```python
from build123d import *

# Parameters (mm, degrees)
F1_DEPTH = 101.6
F2_R     = 2.54
F3_R     = 2.54
F4_R     = 2.54
F5_R     = 2.54
F7_D     = 1.9939


with BuildPart() as f1:
    # F0 (on Top) → F1 (new body)
    with BuildSketch(Plane.XY):
        Polygon((-25.4, 0), (0, 0), (25.4, 0), (25.4, 3.048), (22.6301808, 3.048), (22.6301808, 7.5232392634), (2.54, 7.5232392634), (2.54, 4.2931226644), (0, 4.2931226644), (-2.54, 4.2931226644), (-2.54, 7.5232392634), (-22.6301808, 7.5232392634), (-22.6301808, 3.048), (-25.4, 3.048), align=None)
    extrude(amount=F1_DEPTH)

    # F2
    f2_edges = [f1.edges().sort_by_distance(p)[0] for p in [
        (22.630181, 7.523239, 50.8),
    ]]
    fillet(f2_edges, radius=F2_R)

    # F3
    f3_edges = [f1.edges().sort_by_distance(p)[0] for p in [
        (22.630181, 3.048, 50.8),
    ]]
    fillet(f3_edges, radius=F3_R)

    # F4
    f4_edges = [f1.edges().sort_by_distance(p)[0] for p in [
        (-22.630181, 7.523239, 50.8),
    ]]
    fillet(f4_edges, radius=F4_R)

    # F5
    f5_edges = [f1.edges().sort_by_distance(p)[0] for p in [
        (-22.630181, 3.048, 50.8),
        (-22.630181, 4.983239, 50.8),
    ]]
    fillet(f5_edges, radius=F5_R)

    # F7 (through all)
    with Locations(Plane.XZ):
        with Locations((0, 81.2863707542), (0, 62.5548958778), (0, 40.594484657), (0, 18.223406747)):
            Hole(F7_D / 2)


solid = f1.part
```
Here's how the part is built. I have some questions about the finished solid (model axes, mm). A direction names the side the tool comes from. Give positions to 0.01 mm unless a question says otherwise; leave off trailing zeros. Order: outer loops, then holes, each group sorted by start corner. A loop starts at its lowest first (then second) coordinate and runs counter-clockwise, first axis right, second up. Notation, with made-up numbers: M 26.25,19.25 L 59.25,19.25 A15 ccw 59.25,33.25 Z; hole C 41.25,63.5 d6. An arc over 180 degrees is marked long. Use a Markdown table: item, result. Add a question column.
1. If we mould it in two halves opening along X, with no side actions, what happens to faces 3 (the flat face through (0, 0, 50)), 4 (the cylindrical face through (-21.757, 6.9, 51.511)), 5 (the cylindrical face through (21.795, 6.866, 51.511)), 6 (the cylindrical face through (0.216, 2.177, 61.582))? For each: +X half, -X half, draft (parallel to the pull), parting line (faces both ways), or undercut.
2. I need wall thicknesses on probe 1 along Z at (x, y) = (0, 1.8); probe 2 along Y at (x, z) = (-1.5, 65.5); probe 3 along X at (y, z) = (6, 61.5). Which ranges of each line are inside material? Lowest first, please. Write a range as from..to.
3. Suppose I cut it at B-B (y = 6.25). List the corners of the cut face in (x, z) for me, and give its area (3 significant figures).
4. Suppose I cut it at A-A (x = 0). List the corners of the cut face in (y, z) for me.
5. On a 3-axis mill with a long thin cutter (end or side, diameter ignored), from which of +Z, -Z, +X, -X, +Y, -Y can I reach the whole of each face in a straight line? I mean faces 1 (the cylindrical face through (0.22, 2.18, 17.25)), 2 (the flat face through (2.54, 6, 50)). Say none if no direction works.
6. For pin 1 Ø1.8 at (x, z) = (0, 62.55) entering from +Y; pin 2 Ø3 at (x, z) = (0, 81.29) entering from +Y; pin 3 Ø1 at (y, z) = (5, 36) entering from -X; pin 4 Ø1.6 at (y, z) = (5.5, 70.5) entering from +X, each with a flat end and sliding along its axis, tell me the tip position at first contact or that it passes through.
Results list:
| question | item | result |
|---|---|---|
| 1 | face 3 | draft |
| 1 | face 4 | -X half |
| 1 | face 5 | +X half |
| 1 | face 6 | undercut |
| 2 | probe 1 | z = 0..17.23, 19.22..39.6, 41.59..61.56, 63.55..80.29, 82.28..101.6 |
| 2 | probe 2 | y = 0..4.29 |
| 2 | probe 3 | x = -22.42..-2.54, 2.54..22.42 |
| 3 | outline | M -22.29,0 L -2.54,0 L -2.54,101.6 L -22.29,101.6 Z; M 2.54,0 L 22.29,0 L 22.29,101.6 L 2.54,101.6 Z |
| 3 | area | 4,010 mm² |
| 4 | outline | M 0,0 L 4.29,0 L 4.29,17.23 L 0,17.23 Z; M 0,19.22 L 4.29,19.22 L 4.29,39.6 L 0,39.6 Z; M 0,41.59 L 4.29,41.59 L 4.29,61.56 L 0,61.56 Z; M 0,63.55 L 4.29,63.55 L 4.29,80.29 L 0,80.29 Z; M 0,82.28 L 4.29,82.28 L 4.29,101.6 L 0,101.6 Z |
| 5 | face 1 | +Y, -Y |
| 5 | face 2 | +Z, -Z, +Y |
| 6 | pin 1 | passes through |
| 6 | pin 2 | stops at y = 4.29 |
| 6 | pin 3 | stops at x = -22.84 |
| 6 | pin 4 | stops at x = 22.75 |
